from build123d import *

# Parameters (mm, degrees)
SKETCH1_W           = 200
SKETCH1_H           = 80
BOSS_EXTRUDE1_DEPTH = 3
SKETCH2_R           = 2
CUT_EXTRUDE1_DEPTH  = 108.745069493
FILLET1_R           = 10
CUT_EXTRUDE3_DEPTH  = 108.745069493
SKETCH5_R           = 1.25
CUT_EXTRUDE4_DEPTH  = 108.745069493
SKETCH6_R           = 1.5
CUT_EXTRUDE5_DEPTH  = 108.745069493


with BuildPart() as part:
    # Sketch1 → Boss-Extrude1 (new body)
    with BuildSketch(Plane.XY):
        Rectangle(SKETCH1_W, SKETCH1_H)
    extrude(amount=BOSS_EXTRUDE1_DEPTH)

    # Sketch2 → Cut-Extrude1 (cut, through all)
    with BuildSketch(Plane.XY.offset(3)):
        with Locations((-92, 32)):
            Circle(SKETCH2_R)
        with Locations(Location((-92, -32, 0), (0, 0, 180))):
            Circle(SKETCH2_R)
        with Locations((92, -32)):
            Circle(SKETCH2_R)
        with Locations(Location((92, 32, 0), (0, 0, 180))):
            Circle(SKETCH2_R)
    extrude(amount=-CUT_EXTRUDE1_DEPTH, mode=Mode.SUBTRACT)

    # Fillet1
    fillet1_edges = [part.edges().sort_by_distance(p)[0] for p in [
        (100, -40, 1.5),
        (-100, -40, 1.5),
        (-100, 40, 1.5),
        (100, 40, 1.5),
    ]]
    fillet(fillet1_edges, radius=FILLET1_R)

    # Sketch4 → Cut-Extrude3 (cut, through all)
    with BuildSketch(Plane.XY.offset(3)):
        with BuildLine():
            Line((15, 30), (-15, 30))
            ThreePointArc((-15, 30), (-18, 33), (-15, 36))
            Line((-15, 36), (15, 36))
            ThreePointArc((15, 36), (18, 33), (15, 30))
        make_face()
        with BuildLine():
            Line((15, -30), (-15, -30))
            ThreePointArc((-15, -30), (-18, -33), (-15, -36))
            Line((-15, -36), (15, -36))
            ThreePointArc((15, -36), (18, -33), (15, -30))
        make_face()
    extrude(amount=-CUT_EXTRUDE3_DEPTH, mode=Mode.SUBTRACT)

    # Sketch5 → Cut-Extrude4 (cut, through all)
    with BuildSketch(Plane.XY.offset(3)):
        with Locations((18.55608859, -18.74318761)):
            Circle(SKETCH5_R)
        with Locations((-18.18571173, -18.74318761)):
            Circle(SKETCH5_R)
        with Locations((-18.18571173, 18.63631327)):
            Circle(SKETCH5_R)
        with Locations((18.55608859, 18.63631327)):
            Circle(SKETCH5_R)
    extrude(amount=-CUT_EXTRUDE4_DEPTH, mode=Mode.SUBTRACT)

    # Sketch6 → Cut-Extrude5 (cut, through all)
    with BuildSketch(Plane(origin=(0, 0, 0), x_dir=(-1, 0, 0), z_dir=(0, 0, -1))):
        with Locations((66.5, -15)):
            Circle(SKETCH6_R)
        with Locations((90.5, -15)):
            Circle(SKETCH6_R)
        with Locations((66.5, 15)):
            Circle(SKETCH6_R)
        with Locations((90.5, 15)):
            Circle(SKETCH6_R)
        with Locations((-90.5, -15)):
            Circle(SKETCH6_R)
        with Locations((-66.5, -15)):
            Circle(SKETCH6_R)
        with Locations((-66.5, 15)):
            Circle(SKETCH6_R)
        with Locations((-90.5, 15)):
            Circle(SKETCH6_R)
    extrude(amount=-CUT_EXTRUDE5_DEPTH, mode=Mode.SUBTRACT)


solid = part.part
Verification items for the finished model (mm, model axes). Give positions to 0.01 mm unless a question says otherwise; leave off trailing zeros. Answer as CSV lines item,"result". Start each with the question number.
1. Sectioned sample at A-A (z = 1.9). Count the separate pieces of the cut face and the enclosed holes in it, then the cut area to 3 significant figures.
2. Thickness scan on line 1 (Y direction, x = 66.5, z = 1.05); line 2 (Y direction, x = 90.5, z = 1.8); line 3 (X direction, y = 14, z = 2.75). Record the ranges inside material, lowest first.
3. Depth check by flat-ended pin: pin 1 (2.5 mm diameter, centred on x = -90.5, y = 15, fed in from +Z); pin 2 (4.5 mm diameter, centred on x = -92, y = -32, fed in from -Z). Enter the tip coordinate at first touch or a pass-through.
4. Draft check along X on faces 1 (the face through (-90.153, 31.234, 1.521)), 2 (the face through (96.99, 37.15, 1.52)), 3 (the face through (-1, 1, 3)). Enter one of: pulls with the +X half, pulls with the -X half, needs draft (parallel to the pull), parting line crosses it, or undercut.
Derived:
1,separate pieces,"1"
1,enclosed holes,"18"
1,area,"15,400 mm²"
2,line 1,"-40 to -16.5, -13.5 to 13.5, 16.5 to 40"
2,line 2,"-39.99 to -33.32, -30.68 to -16.5, -13.5 to 13.5, 16.5 to 30.68, 33.32 to 39.99"
2,line 3,"-100 to -91.62, -89.38 to -67.62, -65.38 to 65.38, 67.62 to 89.38, 91.62 to 100"
3,pin 1,"through"
3,pin 2,"z = 0"
4,face 1,"undercut"
4,face 2,"pulls with the +X half"
4,face 3,"needs draft"
